For this review, take the finished solid that the model builds, in its own axes (mm). Coordinates: 2 decimals unless noted, no trailing zeros. Order: outer loops, then holes, each group sorted by start corner. A loop starts at its lowest first (then second) coordinate and runs counter-clockwise, first axis right, second up. Notation, with made-up numbers: (79.25, 76) -> (101.25, 76) arc R17 cw to (101.25, 88) -> close; hole circle Ø1 at (8, -26). An arc over 180 degrees is marked (long way). Answer as a JSON object with one key per item and string values. Group by question number.
1) Add section D-D, the plane x = 44.5. Write out the cut boundary in (y, z), then the cut area to 3 significant figures.
2) Wall thickness on L1, parallel to Z at x = 59.5, y = 3.6; L2, parallel to X at y = 2.95, z = 43.5; L3, parallel to X at y = 3.85, z = 58.5: over which ranges is each line inside the solid? List them lowest first.
3) For pin 1 (3.5 mm diameter, centred on x = -19.74, z = 42.53, fed in from -Y); pin 2 (1 mm diameter, centred on x = 8.5, y = 4, fed in from +Z); pin 3 (2.5 mm diameter, centred on x = -17.5, y = 2, fed in from +Z); pin 4 (1.5 mm diameter, centred on x = 24.5, y = 4.5, fed in from -Z), all flat-tipped, find the tip position at first contact; note any pin that passes through.
4) Add section A-A, the plane z = 62.5. Write out the cut boundary in (x, y), then the cut area to 3 significant figures.
5) Add section C-C, the plane x = -16. Write out the cut boundary in (y, z), then the cut area to 3 significant figures.
6) Add section B-B, the plane y = 2.4. Write out the cut boundary in (x, z).
from build123d import *

# Parameters (mm, degrees)
BOSS_EXTRUDE1_DEPTH = 5
SKETCH4_R           = 2
CUT_EXTRUDE1_DEPTH  = 5
CHAMFER1_SIZE       = 5


with BuildPart() as part:
    # Sketch3 → Boss-Extrude1 (new body)
    with BuildSketch(Plane(origin=(0, 0, 0), x_dir=(1, 0, 0), z_dir=(0, 1, 0))):
        Polygon((-11.092806328, -75.233836931), (-12.882806328, -77.083836936), (-20.742806328, -77.083836936), (-28.592806328, -69.233836936), (-28.592806328, -30.933836936), (-20.742806328, -23.083836936), (-6.592793915, -8.933824523), (1.257206085, -1.083824523), (39.557206085, -1.083824523), (47.407206085, -8.933824523), (69.407218499, -30.933836936), (69.407218499, -69.233836936), (61.507218499, -77.133836936), (53.647218499, -77.133836936), (51.907218499, -75.393836936), (51.907218499, -19.55903866), (47.907218499, -15.55903866), (-7.092806328, -15.55903866), (-11.092806328, -19.55903866), align=None)
    extrude(amount=BOSS_EXTRUDE1_DEPTH)

    # Sketch4 → Cut-Extrude1 (cut)
    with BuildSketch(Plane(origin=(0, 5, 0), x_dir=(1, 0, 0), z_dir=(0, 1, 0))):
        with Locations(Location((-19.742793915, -58.533836936, 0), (0, 0, 270))):
            Circle(SKETCH4_R)
        with Locations(Location((-19.742793915, -42.533836936, 0), (0, 0, 270))):
            Circle(SKETCH4_R)
        with Locations(Location((60.557206085, -41.733836936, 0), (0, 0, 270))):
            Circle(SKETCH4_R)
        with Locations(Location((60.557206085, -58.533836936, 0), (0, 0, 270))):
            Circle(SKETCH4_R)
        with Locations(Location((12.007206085, -9.983836936, 0), (0, 0, 270))):
            Circle(SKETCH4_R)
        with Locations(Location((28.007206085, -9.983836936, 0), (0, 0, 270))):
            Circle(SKETCH4_R)
    extrude(amount=-CUT_EXTRUDE1_DEPTH, mode=Mode.SUBTRACT)

    # Chamfer1
    # the kernel refuses this chamfer: 5 mm, written as the material it takes off along each edge
    with BuildSketch(Plane(origin=(78.499490898, 5, 60.141564537), x_dir=(-0.7068394360706721, 0.027495876610586303, -0.7068394360706748), z_dir=(-0.7071067811865488, 0, 0.7071067811865462))) as chamfer1_piece_1:
        Polygon((CHAMFER1_SIZE * 0.999621916911, CHAMFER1_SIZE * 0.0274958766106), (-CHAMFER1_SIZE * 0.0274958766106, CHAMFER1_SIZE * 0.999621916911), (0, 0), align=None)
    extrude(amount=36.889117022, mode=Mode.SUBTRACT)
    with BuildSketch(Plane(origin=(-11.650533929, 5, 86.176109335), x_dir=(0.7068394360706736, 0.027495876610586337, -0.7068394360706732), z_dir=(-0.7071067811865474, 0, -0.7071067811865477))) as chamfer1_piece_2:
        Polygon((CHAMFER1_SIZE * 0.999621916911, CHAMFER1_SIZE * 0.0274958766106), (-CHAMFER1_SIZE * 0.0274958766106, CHAMFER1_SIZE * 0.999621916911), (0, 0), align=None)
    extrude(amount=36.818406344, mode=Mode.SUBTRACT)
    with BuildSketch(Plane(origin=(-28.592806328, 5, 82.092251876), x_dir=(0.9996219169112968, 0.027495876610586317, 0), z_dir=(0, 0, -1)), Plane(origin=(-11.601208855, 5, 1.083824523), x_dir=(3.4424184920964096e-15, 0.027495876610586317, 0.9996219169112968), z_dir=(1, 0, 0)), Plane(origin=(69.407218499, 5, 18.075421996), x_dir=(-0.9996219169112968, 0.027495876610586282, 0), z_dir=(0, 0, 1))) as chamfer1_piece_3:
        Polygon((CHAMFER1_SIZE * 0.999621916911, CHAMFER1_SIZE * 0.0274958766106), (-CHAMFER1_SIZE * 0.0274958766106, CHAMFER1_SIZE * 0.999621916911), (0, 0), align=None)
    extrude(amount=64.01682988, mode=Mode.SUBTRACT)
    with BuildSketch(Plane(origin=(-37.685078728, 5, 40.026109335), x_dir=(0.7068394360706731, 0.027495876610586303, 0.7068394360706738), z_dir=(0.7071067811865479, 0, -0.7071067811865474)), Plane(origin=(30.464933686, 5, -8.008447877), x_dir=(-0.7068394360706771, 0.027495876610586313, 0.70683943607067), z_dir=(0.707106781186544, 0, 0.707106781186551))) as chamfer1_piece_4:
        Polygon((CHAMFER1_SIZE * 0.999621916911, CHAMFER1_SIZE * 0.0274958766106), (-CHAMFER1_SIZE * 0.0274958766106, CHAMFER1_SIZE * 0.999621916911), (0, 0), align=None)
    extrude(amount=67.931122272, mode=Mode.SUBTRACT)


solid = part.part
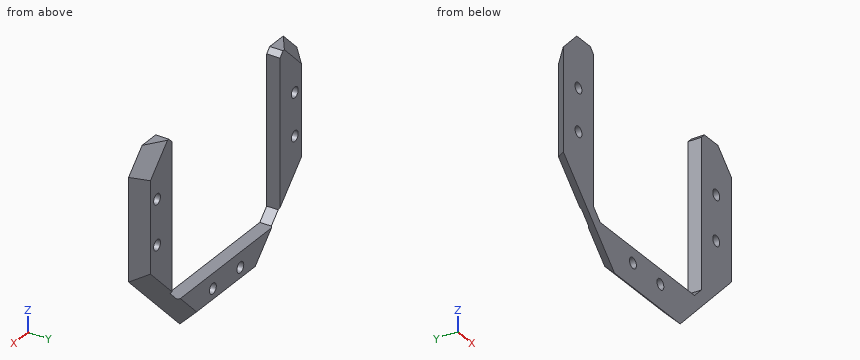
Output values:
{
 "1": {"outline": "(0, 6.03) -> (5, 13.1) -> (5, 15.56) -> (0, 15.56) -> close", "area": "30.0 mm²"},
 "2": {"L1": "z = 26.12 to 40.04, 43.43 to 56.84, 60.23 to 74.05", "L2": "x = -25.64 to -21.49, -17.99 to -11.09, 51.91 to 59.62, 61.5 to 66.46", "L3": "x = -24.74 to -21.74, -17.74 to -11.09, 51.91 to 58.56, 62.56 to 65.56"},
 "3": {"pin 1": "passes through", "pin 2": "stops at z = 15.56", "pin 3": "stops at z = 77.08", "pin 4": "stops at z = 4.83"},
 "4": {"outline": "(-28.59, 0) -> (-11.09, 0) -> (-11.09, 5) -> (-23.59, 5) -> close; (51.91, 0) -> (69.41, 0) -> (64.41, 5) -> (51.91, 5) -> close", "area": "150 mm²"},
 "5": {"outline": "(0, 18.34) -> (5, 25.41) -> (5, 74.76) -> (3.35, 77.08) -> (0, 77.08) -> close", "area": "274 mm²"},
 "6": {"outline": "(-26.19, 31.93) -> (2.25, 3.48) -> (38.56, 3.48) -> (67.01, 31.93) -> (67.01, 68.24) -> (58.11, 77.13) -> (53.65, 77.13) -> (51.91, 75.39) -> (51.91, 19.56) -> (47.91, 15.56) -> (-7.09, 15.56) -> (-11.09, 19.56) -> (-11.09, 75.23) -> (-12.88, 77.08) -> (-17.35, 77.08) -> (-26.19, 68.24) -> close; hole circle Ø4 at (-19.74, 42.53); hole circle Ø4 at (-19.74, 58.53); hole circle Ø4 at (12.01, 9.98); hole circle Ø4 at (28.01, 9.98); hole circle Ø4 at (60.56, 41.73); hole circle Ø4 at (60.56, 58.53)"}
}
